from build123d import *

# Parameters (mm, degrees)
F_70X45X5_1_DEPTH   = 2230
CUT_EXTRUDE_1_REACH = 2252.827
SKETCH_12_R         = 7
CUT_EXTRUDE_2_REACH = 2252.827
SKETCH_13_R         = 7
CHAMFER_1_SIZE      = 30
CHAMFER_2_SIZE      = 30


with BuildPart() as part:
    # 草图11 → 不等边角钢 70X45X5(1) (new body)
    with BuildSketch(Plane(origin=(1115, 1931.236650439, 0), x_dir=(0.86602540378444, -0.49999999999999784, 0), z_dir=(-0.49999999999999784, -0.86602540378444, 0))):
        with BuildLine():
            Line((0, 70), (0, 0))
            Line((0, 0), (45, 0))
            Line((45, 0), (45, 3.33))
            ThreePointArc((45, 3.33), (44.510868325, 4.510868325), (43.33, 5))
            Line((43.33, 5), (12.5, 5))
            ThreePointArc((12.5, 5), (7.196699141, 7.196699141), (5, 12.5))
            Line((5, 12.5), (5, 68.33))
            ThreePointArc((5, 68.33), (4.510868325, 69.510868325), (3.33, 70))
            Line((3.33, 70), (0, 70))
        make_face()
    extrude(amount=F_70X45X5_1_DEPTH)

    # 草图12 → 切除-拉伸1 (cut, up to next)
    with BuildSketch(Plane(origin=(0, 0, 0), x_dir=(0, 0, 1), z_dir=(-0.86602540378444, 0.49999999999999784, 0)), mode=Mode.PRIVATE) as cut_extrude_1_sk1:
        with Locations(Location((40, 30, 0), (0, 0, 270))):
            Circle(SKETCH_12_R)
    cut_extrude_1_tool1 = extrude(cut_extrude_1_sk1.sketch, amount=-CUT_EXTRUDE_1_REACH, mode=Mode.PRIVATE) & part.part
    # 草图12 → 切除-拉伸1 (cut, up to next)
    with BuildSketch(Plane(origin=(0, 0, 0), x_dir=(0, 0, 1), z_dir=(-0.86602540378444, 0.49999999999999784, 0)), mode=Mode.PRIVATE) as cut_extrude_1_sk2:
        with Locations(Location((40, 110, 0), (0, 0, 270))):
            Circle(SKETCH_12_R)
    cut_extrude_1_tool2 = extrude(cut_extrude_1_sk2.sketch, amount=-CUT_EXTRUDE_1_REACH, mode=Mode.PRIVATE) & part.part
    add(cut_extrude_1_tool1.solids().sort_by_distance((15, 25.980762, 40))[0], mode=Mode.SUBTRACT)
    add(cut_extrude_1_tool2.solids().sort_by_distance((55, 95.262794, 40))[0], mode=Mode.SUBTRACT)

    # 草图13 → 切除-拉伸2 (cut, up to next)
    with BuildSketch(Plane(origin=(0, 0, 0), x_dir=(0, 0, 1), z_dir=(-0.86602540378444, 0.49999999999999784, 0)), mode=Mode.PRIVATE) as cut_extrude_2_sk1:
        with Locations(Location((40.004723234, 2120, 0), (0, 0, 270))):
            Circle(SKETCH_13_R)
    cut_extrude_2_tool1 = extrude(cut_extrude_2_sk1.sketch, amount=-CUT_EXTRUDE_2_REACH, mode=Mode.PRIVATE) & part.part
    # 草图13 → 切除-拉伸2 (cut, up to next)
    with BuildSketch(Plane(origin=(0, 0, 0), x_dir=(0, 0, 1), z_dir=(-0.86602540378444, 0.49999999999999784, 0)), mode=Mode.PRIVATE) as cut_extrude_2_sk2:
        with Locations(Location((40.004723234, 2200, 0), (0, 0, 270))):
            Circle(SKETCH_13_R)
    cut_extrude_2_tool2 = extrude(cut_extrude_2_sk2.sketch, amount=-CUT_EXTRUDE_2_REACH, mode=Mode.PRIVATE) & part.part
    add(cut_extrude_2_tool1.solids().sort_by_distance((1060, 1835.973856, 40.004723))[0], mode=Mode.SUBTRACT)
    add(cut_extrude_2_tool2.solids().sort_by_distance((1100, 1905.255888, 40.004723))[0], mode=Mode.SUBTRACT)

    # 倒角1
    # the kernel refuses this chamfer: 30 mm, written as the material it takes off along each edge
    with BuildSketch(Plane(origin=(1184.698148536, 1890.99640562, 70), x_dir=(-0.49981095845564616, -0.8656979742248816, 0.02749587661058632), z_dir=(-0.86602540378444, 0.49999999999999784, 0))) as chamfer_1_piece_1:
        Polygon((CHAMFER_1_SIZE * 0.999621916911, -CHAMFER_1_SIZE * 0.0274958766106), (-CHAMFER_1_SIZE * 0.0274958766106, -CHAMFER_1_SIZE * 0.999621916911), (0, 0), align=None)
    extrude(amount=157.630979278, mode=Mode.SUBTRACT)

    # 倒角2
    # the kernel refuses this chamfer: 30 mm, written as the material it takes off along each edge
    with BuildSketch(Plane(origin=(69.698148536, -40.240244819, 70), x_dir=(-0.013747938305293054, -0.023812127644090075, -0.9996219169112966), z_dir=(-0.86602540378444, 0.49999999999999784, 0))) as chamfer_2_piece_1:
        Polygon((CHAMFER_2_SIZE * 0.999621916911, -CHAMFER_2_SIZE * 0.0274958766106), (-CHAMFER_2_SIZE * 0.0274958766106, -CHAMFER_2_SIZE * 0.999621916911), (0, 0), align=None)
    extrude(amount=157.630979278, mode=Mode.SUBTRACT)


solid = part.part
CAD build for the part. Positions are in the model's coordinates, mm. A direction names the side the tool comes from. Coordinates: 2 decimals unless noted, no trailing zeros. Use a Markdown table: item, result. Add a question column.
Item 1: Drill centre lines: L1, parallel to Z at x = 198, y = 297.5; L2, parallel to Y at x = 932.5, z = 27; L3, parallel to X at y = 1640, z = 30.5. Where is each one in solid material? Low to high. Write a range as from..to.
Item 2: Flat gauge pins, fed straight in: pin 1 (12 mm diameter, centred on y = 710, z = 31, fed in from -X); pin 2 (10 mm diameter, centred on y = 341, z = 48.5, fed in from +X); pin 3 (12 mm diameter, centred on x = 374, z = 23.5, fed in from -Y). Where does each tip first touch, or does it go through?
Item 3: 3-axis set-ups, long thin cutter, end or side, ignore diameter. For faces 1 (the face through (567, 978, 70)), 2 (the face through (590, 965, 5)): which of +Z, -Z, +X, -X, +Y, -Y reach the whole face in a straight line?
Numbers:
| question | item | result |
|---|---|---|
| 1 | L1 | 0..5 |
| 1 | L2 | 1605.14..1615.14 |
| 1 | L3 | 946.85..952.63 |
| 2 | pin 1 | x = 406.45 |
| 2 | pin 2 | x = 205.54 |
| 2 | pin 3 | y = 627.39 |
| 3 | face 1 | +Z, +X, -X, +Y, -Y |
| 3 | face 2 | +Z, +X, -Y |
